```python
from build123d import *

# Parameters (mm, degrees)
SKETCH1_R           = 120
BOSS_EXTRUDE1_DEPTH = 20
SKETCH2_R           = 60
BOSS_EXTRUDE2_DEPTH = 100
CUT_EXTRUDE1_DEPTH  = 121
BOSS_EXTRUDE3_DEPTH = 25
BOSS_EXTRUDE4_START = -40
SKETCH5_R           = 25
BOSS_EXTRUDE4_DEPTH = 50
SKETCH6_R           = 15
CUT_EXTRUDE2_DEPTH  = 51
CIRPATTERN1_COUNT   = 3
FILLET2_R           = 10


with BuildPart() as part:
    # Sketch1 → Boss-Extrude1 (new body)
    with BuildSketch(Plane(origin=(0, 0, 0), x_dir=(1, 0, 0), z_dir=(0, 1, 0))):
        with Locations(Location((0, 0, 0), (0, 0, 270))):  # turned: the seam where the file's is
            Circle(SKETCH1_R)
    extrude(amount=BOSS_EXTRUDE1_DEPTH)

    # Sketch2 → Boss-Extrude2 (add)
    with BuildSketch(Plane.XZ):
        with Locations(Location((0, 0, 0), (0, 0, 270))):  # turned: the seam where the file's is
            Circle(SKETCH2_R)
    extrude(amount=BOSS_EXTRUDE2_DEPTH)

    # Sketch3 → Cut-Extrude1 (cut, through all)
    with BuildSketch(Plane(origin=(0, 20, 0), x_dir=(1, 0, 0), z_dir=(0, 1, 0))):
        with BuildLine():
            Line((27.549954628, 5), (36, 5))
            Line((36, 5), (36, -5))
            Line((36, -5), (27.549954628, -5))
            ThreePointArc((27.549954628, -5), (-28, 0), (27.549954628, 5))
        make_face()
    extrude(amount=-CUT_EXTRUDE1_DEPTH, mode=Mode.SUBTRACT)

    # Sketch4 → Boss-Extrude3 (add, symmetric)
    with BuildSketch(Plane.XY):
        Polygon((-45.582672643, -70), (-86, -70), (-176, -160), (-211, -160), (-211, -190), (-163.573593129, -190), (-73.573593129, -100), (-45.582672643, -100), align=None)
    boss_extrude3 = extrude(amount=BOSS_EXTRUDE3_DEPTH, both=True)

    # Sketch5 → Boss-Extrude4 (add)
    with BuildSketch(Plane(origin=(0, -160, 0), x_dir=(1, 0, 0), z_dir=(0, 1, 0)).offset(BOSS_EXTRUDE4_START)):
        with Locations(Location((-211, 0, 0), (0, 0, 270))):  # turned: the seam where the file's is
            Circle(SKETCH5_R)
    boss_extrude4 = extrude(amount=BOSS_EXTRUDE4_DEPTH)

    # Sketch6 → Cut-Extrude2 (cut, through all)
    with BuildSketch(Plane(origin=(0, -150, 0), x_dir=(1, 0, 0), z_dir=(0, 1, 0))):
        with Locations(Location((-211, 0, 0), (0, 0, 270))):  # turned: the seam where the file's is
            Circle(SKETCH6_R)
    cut_extrude2 = extrude(amount=-CUT_EXTRUDE2_DEPTH, mode=Mode.SUBTRACT)

    # CirPattern1: Boss-Extrude3, Boss-Extrude4, Cut-Extrude2 ×3 about axis
    cirpattern1_axis = Axis((0, 0, 0), (0, 1, 0))
    add([boss_extrude3.rotate(cirpattern1_axis, i * 360 / CIRPATTERN1_COUNT) for i in range(1, CIRPATTERN1_COUNT)])
    add([boss_extrude4.rotate(cirpattern1_axis, i * 360 / CIRPATTERN1_COUNT) for i in range(1, CIRPATTERN1_COUNT)])
    add([cut_extrude2.rotate(cirpattern1_axis, i * 360 / CIRPATTERN1_COUNT) for i in range(1, CIRPATTERN1_COUNT)], mode=Mode.SUBTRACT)

    # Fillet2
    fillet2_edges = [part.edges().sort_by_distance(p)[0] for p in [
        (0, 0, 60),
    ]]
    fillet(fillet2_edges, radius=FILLET2_R)


solid = part.part
```
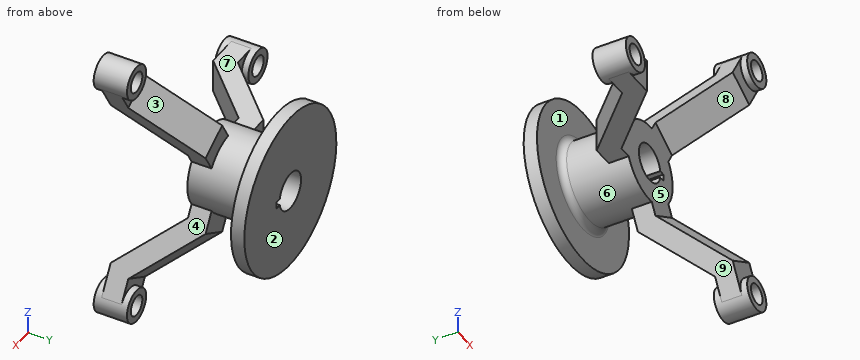
Part model, mm, in its own coordinate system. Face numbers are marked on the shaded views. A direction names the side the tool comes from. Coordinates: 2 decimals unless noted, no trailing zeros. Loops run counter-clockwise (first coordinate to the right, second up) from the corner with the lowest first, then second, coordinate; pieces in that order, holes last. Notation, with made-up numbers: (16, 36.5) - (48, 36.5) arc R17 cw to (48, 47.5) - close; hole circle Ø11 at (64, 10). An arc over 180 degrees is marked (long way). Write item = value, one per line. Start each with the question number.
Item 1: Mould opens along Y. For the marked faces 1, 2, 3 and 4 say: released by +Y, released by -Y, zero draft, split by the parting line, or undercut.
Item 2: 3-axis set-ups, long thin cutter, end or side, ignore diameter. For the marked faces 5, 6, 7, 8 and 9: which of +Z, -Z, +X, -X, +Y, -Y reach the whole face in a straight line?
Item 3: Cut at A-A, the plane z = 0. Give the cut face in (x, y), and give its area (3 significant figures).
Item 4: Wall check: L1, parallel to X at y = -71, z = 0; L2, parallel to X at y = -45.5, z = 0; L3, parallel to Z at x = 105, y = -185. Give the ranges that are in metal, low to high. Write a range as from..to.
Item 5: Flat gauge pins, fed straight in: pin 1 Ø25 at (x, z) = (102.5, 180.5) entering from +Y; pin 2 Ø1 at (x, y) = (39.5, -63.5) entering from -Z; pin 3 Ø11 at (y, z) = (-22.5, 0.5) entering from -X. Where does each tip first touch, or does it go through?
Item 6: Cut at D-D, the plane y = -79. Give the cut face in (x, z), and give its area (3 significant figures).
Item 7: Cut at C-C, the plane y = -118.5. Give the cut face in (x, z).
Item 8: Cut at B-B, the plane x = 0. Give the cut face in (y, z), and give its area (3 significant figures).
The answers:
q1.face_1 = undercut
q1.face_2 = released by +Y
q1.face_3 = undercut
q1.face_4 = zero draft
q2.face_5 = -Y
q2.face_6 = none
q2.face_7 = +Z, -X, -Y
q2.face_8 = -X, -Y
q2.face_9 = -Z, -X, -Y
q3.outline = (-236, -200) - (-226, -200) - (-226, -150) - (-236, -150) - close; (-196, -200) - (-186, -200) - (-186, -190) - (-163.57, -190) - (-73.57, -100) - (-28, -100) - (-28, 20) - (-120, 20) - (-120, 0) - (-70, 0) arc R10 cw to (-60, -10) - (-60, -70) - (-86, -70) - (-176, -160) - (-186, -160) - (-186, -150) - (-196, -150) - close; (36, -100) - (60, -100) - (60, -10) arc R10 cw to (70, 0) - (120, 0) - (120, 20) - (36, 20) - close
q3.area = 15,100 mm2
q4.L1 = -87..-28, 36..60
q4.L2 = -60..-28, 36..60
q4.L3 = -207.73..-197.72, -167.74..-131.87, 131.87..167.74, 197.72..207.73
q5.pin_1 = -150
q5.pin_2 = -45.6
q5.pin_3 = -60
q6.outline = (-95, -25) - (-54.54, -25) arc R60 ccw to (5.62, -59.74) - (25.85, -94.77) - (69.15, -69.77) - (48.92, -34.74) arc R60 ccw to (48.92, 34.74) - (69.15, 69.77) - (25.85, 94.77) - (5.62, 59.74) arc R60 ccw to (-54.54, 25) - (-95, 25) - close; hole (27.55, -5) - (36, -5) - (36, 5) - (27.55, 5) arc R28 ccw (long way) to start
q6.area = 14,300 mm2
q7.outline = (-134.5, -25) - (-92.07, -25) - (-92.07, 25) - (-134.5, 25) - close; (24.39, -92.24) - (45.6, -128.98) - (88.9, -103.98) - (67.69, -67.24) - close; (24.39, 92.24) - (67.69, 67.24) - (88.9, 103.98) - (45.6, 128.98) - close
q8.outline = (-100, -60) - (-10, -60) arc R10 cw to (0, -70) - (0, -120) - (20, -120) - (20, -28) - (-100, -28) - close; (-100, 28) - (20, 28) - (20, 120) - (0, 120) - (0, 70) arc R10 cw to (-10, 60) - (-100, 60) - close
q8.area = 10,100 mm2
